Autodesk Inventor part; units mm, degrees
ref_plane "YZ Plane" through (0, 0, 0) normal (1, 0, 0) x (0, 1, 0)
ref_plane "XZ Plane" through (0, 0, 0) normal (0, 1, 0) x (-1, 0, 0)
ref_plane "XY Plane" through (0, 0, 0) normal (0, 0, 1) x (1, 0, 0)
sketch "Sketch1" plane through (0, 0, 0) normal (0, 1, 0) x (-1, 0, 0)
  line L0 (0, -35) -> (4, -35)
  line L1 (-48, 0) -> (-48, -35)
  line L2 (-48, -24.7754) -> (-48, -13.3333)
  line L3 (-48, -35) -> (-52, -35)
  line L4 (-52, -35) -> (-52, -33)
  line L5 (-52, -33) -> (-124, -33)
  line L6 (4, -35) -> (4, -33)
  line L7 (4, -33) -> (76, -33)
  line L8 (0, 0) -> (0, -35)
  line L9 (0, -96.6) -> (0, 47.6)
  line L10 (0, 0) -> (-48, 0)
  line L11 (76, -33) -> (76, 27)
  line L12 (76, 27) -> (-124, 27)
  line L13 (-124, 27) -> (-124, -33)
  line L14 (-24, 27) -> (-24, -76) construction
  dimension "d0" = 35
  dimension "d1" = 35
  dimension "d3" = 4
  dimension "d4" = 2
  dimension "d6" = 48
  dimension "d13" = 60
  dimension "d20" = 100
extrude "Extrusion1" add sketch "Sketch1" along normal blind 5
sketch "Sketch2" plane through (0, 5, 0) normal (0, 1, 0) x (1, 0, 0)
  line L0 (-4, 35) -> (-4, 33)
  line L1 (0, 0) -> (0, 35)
  line L2 (-4, 35) -> (0, 35)
  line L3 (0, 35) -> (0, 25)
  line L4 (0, 25) -> (-4, 25)
  line L5 (-4, 25) -> (-4, 35)
  line L6 (52, 35) -> (48, 35)
  line L7 (52, 35) -> (48, 35)
  line L8 (48, 35) -> (48, 25)
  line L9 (48, 25) -> (52, 25)
  line L10 (52, 25) -> (52, 35)
  dimension "d21" = 10
  dimension "d22" = 10
extrude "Extrusion2" add sketch "Sketch2" along normal blind 10
sketch "Sketch3" plane through (-4, 0, -35) normal (-1, 0, 0) x (0, 0, 1)
  circle A0 centre (5, 10) radius 2
  line L0 (0, 0) -> (0, 15)
  line L1 (0, 15) -> (10, 15)
  point P0 (35, 0)
  dimension "d25" = 4
  dimension "d26" = 5
  dimension "d27" = 5
extrude "Extrusion3" cut sketch "Sketch3" against normal through all
sketch "Sketch7" plane through (0, 5, 0) normal (0, 1, 0) x (1, 0, 0)
  line L0 (-4, 33) -> (-76, 33)
  line L1 (-76, -27) -> (124, -27)
  line L2 (-76, 33) -> (-66, 33)
  line L3 (-66, 33) -> (-66, -27)
  line L4 (-66, -27) -> (-76, -27)
  line L5 (-76, -27) -> (-76, 33)
  line L6 (124, 33) -> (114, 33)
  line L7 (114, 33) -> (114, -27)
  line L8 (114, -27) -> (124, -27)
  line L9 (124, -27) -> (124, 33)
  point P0 (0, 0)
  dimension "d42" = 10
  dimension "d43" = 10
  dimension "d67" = 190
extrude "Extrusion7" add sketch "Sketch7" along normal blind 45
sketch "Sketch8" plane through (0, 50, 0) normal (0, 1, 0) x (1, 0, 0)
  line L0 (-76, -27) -> (-76, 33)
  line L1 (124, -27) -> (124, 33)
  line L2 (-76, -27) -> (124, -27)
  line L3 (124, -27) -> (124, 33)
  line L4 (124, 33) -> (-76, 33)
  line L5 (-76, 33) -> (-76, -27)
extrude "Extrusion8" add sketch "Sketch8" along normal blind 10
sketch "Sketch9" plane through (0, 50, 0) normal (0, -1, 0) x (1, 0, 0)
  line L0 (48, -35) -> (48, -25)
  line L1 (0, 0) -> (0, -35)
  line L2 (0, -33) -> (48, -33)
  line L3 (48, -33) -> (48, -18)
  line L4 (48, -18) -> (0, -18)
  line L5 (0, -18) -> (0, -33)
  dimension "d50" = 15
extrude "Extrusion9" cut sketch "Sketch9" against normal blind 2.5
sketch "Sketch10" plane through (0, 52.5, 0) normal (0, -1, 0) x (1, 0, 0)
  line L0 (0, -25.5) -> (11, -25.5)
  line L1 (0, 0) -> (0, -35)
  circle A0 centre (11, -25.5) radius 2
  line L2 (48, -18) -> (48, -33)
  line L3 (48, -25.5) -> (37, -25.5)
  circle A1 centre (37, -25.5) radius 2
  line L4 (48, -33) -> (0, -33)
  dimension "d55" = 11
  dimension "d57" = 4
  dimension "d58" = 11
  dimension "d68" = 7.5
extrude "Extrusion10" cut sketch "Sketch10" against normal through all
sketch "Sketch12" plane through (0, 50, 0) normal (0, -1, 0) x (1, 0, 0)
  circle A0 centre (-27.5, 7) radius 10.95
  circle A1 centre (75.5, 7) radius 10.95
  point P0 (0, 0)
  dimension "d64" = 21.9
extrude "Extrusion12" cut sketch "Sketch12" against normal blind 7
sketch "Sketch16" plane through (-27.5, 57, 7) normal (0, -1, 0) x (1, 0, 0)
  circle A0 centre (0, 0) radius 6
  circle A1 centre (103, 0) radius 10.95
  circle A2 centre (103, 0) radius 6
  point P0 (27.5, -7)
  dimension "d88" = 12
extrude "Extrusion15" cut sketch "Sketch16" against normal through all contours A0 | A2
sketch "Sketch17" plane through (0, 60, 0) normal (0, 1, 0) x (1, 0, 0)
  circle A0 centre (75.5, -7) radius 6
  line L0 (75.5, -7) -> (75.5, 1.4)
  line L1 (60.5, 1.4) -> (90.5, 1.4)
  line L2 (90.5, 1.4) -> (90.5, 11.4)
  line L3 (90.5, 11.4) -> (60.5, 11.4)
  line L4 (60.5, 11.4) -> (60.5, 1.4)
  circle A1 centre (75.5, -7) radius 10.95
  circle A2 centre (-27.5, -7) radius 6
  line L5 (75.5, -7) -> (-27.5, -7)
  line L6 (24, -7) -> (24, -1)
  line L7 (-12.5, 1.4) -> (-42.5, 1.4)
  line L8 (-42.5, 1.4) -> (-42.5, 11.4)
  line L9 (-42.5, 11.4) -> (-12.5, 11.4)
  line L10 (-12.5, 11.4) -> (-12.5, 1.4)
  point P0 (0, 0)
  dimension "d91" = 8.4
  dimension "d92" = 30
  dimension "d93" = 10
extrude "Extrusion16" add sketch "Sketch17" along normal blind 40 contours L1 A1 | L1 L4 L3 L2 A1 | L7 L8 L9 L10
sketch "Sketch18" plane through (60.5, 60, -1.4) normal (0, 0, 1) x (1, 0, 0)
  circle A0 centre (4, 20) radius 2
  line L0 (-136.5, 0) -> (63.5, 0)
  line L1 (0, 0) -> (0, 40)
  line L2 (0, 0) -> (30, 0)
  line L3 (15, 0) -> (15, 6)
  circle A1 centre (26, 20) radius 2
  point P0 (-60.5, -60)
  dimension "d96" = 20
  dimension "d97" = 4
  dimension "d98" = 4
extrude "Extrusion17" cut sketch "Sketch18" against normal through all
sketch "Sketch19" plane through (-42.5, 60, -1.4) normal (0, 0, 1) x (1, 0, 0)
  line L0 (-33.5, 0) -> (166.5, 0)
  line L1 (133, 0) -> (-1, 0)
  line L2 (66, 0) -> (66, 10)
  circle A0 centre (107, 20) radius 2
  circle A1 centre (107, 20) radius 2
  circle A2 centre (129, 20) radius 2
  circle A3 centre (129, 20) radius 2
  circle A4 centre (25, 20) radius 2
  circle A5 centre (3, 20) radius 2
  point P0 (42.5, -60)
extrude "Extrusion18" cut sketch "Sketch19" against normal through all contours A4 | A5
equation "\"d1\" = d0"
properties part number "upper part shooter_3DPrint"
Here's how the part is built. I have some questions about the finished solid (model axes, mm). A direction names the side the tool comes from. Round coordinates to 2 decimals unless told otherwise and drop trailing zeros. Write each loop counter-clockwise with the first axis right and the second up, starting at its lowest first coordinate (ties: lowest second). Pieces come first, ordered by that corner, then holes.
1. Suppose I cut it at A-A (x = 46). List the corners of the cut face in (y, z) for me, and give its area (4 significant figures).
2. If we mould it in two halves opening along Y, with no side actions, what happens to faces 4 (the flat face through (-76, 30, -3)), 5 (the flat face through (75, 100, -6)), 6 (the flat face through (24, 52.5, -25)), 7 (the flat face through (50, 10, -25))? For each: released by +Y, released by -Y, zero draft, split by the parting line, or undercut.
3. For faces 1 (the flat face through (24, 2, 0)), 2 (the flat face through (-12.5, 80, -6)), 3 (the flat face through (114, 27, -3)), which set-ups out of +Z, -Z, +X, -X, +Y, -Y let a thin tool reach every point of the face, with its end or its side?
4. Will these pins go through, and if not, where does the flat tip stop? pin 1 Ø5 at (x, z) = (14.5, -3.5) entering from +Y; pin 2 Ø6.5 at (x, y) = (-17.5, 80) entering from +Z; pin 3 Ø11 at (y, z) = (76.5, -5) entering from -X.
5. Suppose I cut it at D-D (y = 27.5). List the corners of the cut face in (x, z) for me.
6. I need wall thicknesses on L1, parallel to Y at x = 49.5, z = -30; L2, parallel to Y at x = 86.5, z = -4.75; L3, parallel to Y at x = -11.5, z = -8. Which ranges of each line are inside material? Lowest first, please.
7. Suppose I cut it at C-C (x = 11). List the corners of the cut face in (y, z) for me, and give its area (4 significant figures).
8. Suppose I cut it at B-B (z = -30). List the corners of the cut face in (x, y) for me.
Answer sheet:
1. outline: (0, 0) - (5, 0) - (5, 27) - (0, 27) - close; (50, -18) - (52.5, -18) - (52.5, -33) - (60, -33) - (60, 27) - (50, 27) - close
1. area: 697.5 mm2
2. face 4: zero draft
2. face 5: released by +Y
2. face 6: released by -Y
2. face 7: undercut
3. face 1: -Z, -Y
3. face 2: +Z, -Z, +Y
3. face 3: +Z, -Z
4. pin 1: stops at y = 60
4. pin 2: stops at z = -1.4
4. pin 3: stops at x = -42.5
5. outline: (-76, -33) - (-66, -33) - (-66, 27) - (-76, 27) - close; (114, -33) - (124, -33) - (124, 27) - (114, 27) - close
6. L1: y = 0 to 8, 12 to 15, 50 to 60
6. L2: y = 0 to 5, 50 to 78, 82 to 100
6. L3: y = 0 to 5, 50 to 60
7. outline: (0, 0) - (5, 0) - (5, 27) - (0, 27) - close; (50, -18) - (52.5, -18) - (52.5, -23.5) - (60, -23.5) - (60, 27) - (50, 27) - close; (52.5, -33) - (60, -33) - (60, -27.5) - (52.5, -27.5) - close
7. area: 667.5 mm2
8. outline: (-76, 0) - (0, 0) - (0, 8) - (-4, 8) - (-4, 5) - (-66, 5) - (-66, 50) - (0, 50) - (0, 52.5) - (48, 52.5) - (48, 50) - (114, 50) - (114, 5) - (52, 5) - (52, 8) - (48, 8) - (48, 0) - (124, 0) - (124, 60) - (-76, 60) - close; (-4, 12) - (0, 12) - (0, 15) - (-4, 15) - close; (48, 12) - (52, 12) - (52, 15) - (48, 15) - close
